Geometry: final body of the model. Coordinates: model frame, mm. Face numbers are marked on the shaded views. A direction names the side the tool comes from. Round coordinates to 2 decimals unless told otherwise and drop trailing zeros. Loops run counter-clockwise (first coordinate to the right, second up) from the corner with the lowest first, then second, coordinate; pieces in that order, holes last. Notation, with made-up numbers: (19.25, -37.75) - (50.25, -37.75) arc R16 cw to (50.25, -11.75) - close; hole circle Ø3 at (59.5, 2.5). An arc over 180 degrees is marked (long way). Answer as a JSON object with one key per item and string values. Group by question number.
Item 1: Section C-C (x = 111). Return the cut outline in (y, z), plus the area to 3 significant figures.
Item 2: Reachability of the marked faces 1 and 2 from +Z, -Z, +X, -X, +Y, -Y: full face, straight path, thin tool, end or side. Return the list, or none.
Item 3: Section D-D (y = 41). Return the cut outline in (x, z), plus the area to 3 significant figures.
Item 4: Section B-B (y = 10.5). Return the cut outline in (x, z), plus the area to 3 significant figures.
Item 5: Draft query along X for the marked faces 3, 4, 5 and 6. Return one class per face: released by +X, released by -X, zero draft, split by the parting line, or undercut.
Item 6: Line query: line 1 (Z direction, x = 30, y = 2); line 2 (Y direction, x = 100.5, z = 15.5); line 3 (X direction, y = 50, z = 6.5). Output: solid intervals per line, ascending.
Item 7: Section A-A (z = 10). Return the cut outline in (x, y).
Item 8: First-contact query: pin 1 (1.6 mm diameter, centred on x = 36, z = 15, fed in from +Y); pin 2 (2 mm diameter, centred on x = 115, y = 55.5, fed in from +Z); pin 3 (3 mm diameter, centred on x = 36, z = 15, fed in from -Y). Flat tips, straight axial feed; report the tip coordinate or a pass-through.
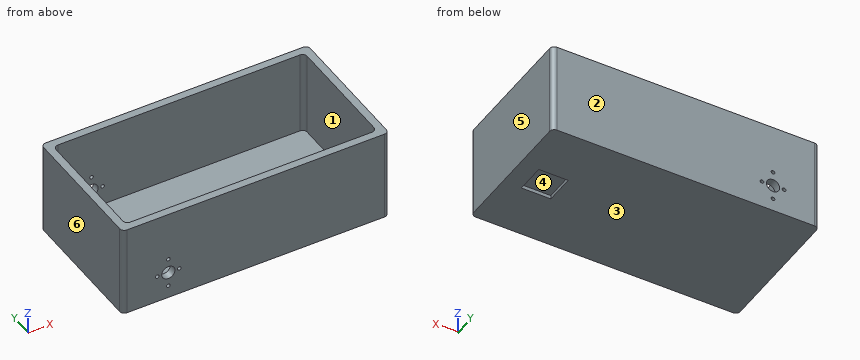
Autodesk Fusion 360 part; units mm, degrees
sketch "Skizze1" plane through (0, 0, 0) normal (0, 0, 1) x (1, 0, 0)
  line L0 (5, 0) -> (150, 0)
  line L1 (150, 0) -> (150, 75)
  line L2 (150, 75) -> (5, 75)
  line L3 (5, 75) -> (5, 0)
extrude "Extrusion1" add sketch "Skizze1" along normal blind 50
shell "Schale1" thickness 4.2 removed faces 1 at (53.3333, 50, 50)
fillet "Abrundung1" radius 2.5 1 edges at (5, 0, 25)
fillet "Abrundung2" radius 2.5 1 edges at (9.2, 4.2, 27.1)
fillet "Abrundung3" radius 2.5 1 edges at (9.2, 70.8, 27.1)
fillet "Abrundung4" radius 2.5 1 edges at (5, 75, 25)
fillet "Abrundung5" radius 2.5 1 edges at (150, 75, 25)
fillet "Abrundung6" radius 2.5 1 edges at (145.8, 70.8, 27.1)
fillet "Abrundung7" radius 2.5 1 edges at (145.8, 4.2, 27.1)
fillet "Abrundung8" radius 2.5 1 edges at (150, 0, 25)
sketch "Skizze2" plane through (0, 75, 0) normal (0, 1, 0) x (-1, 0, 0)
  line L0 (-147.5, 50) -> (-147.5, 0)
  line L1 (-147.5, 0) -> (-7.5, 0)
  line L2 (-7.5, 0) -> (-7.5, 50)
  line L3 (-7.5, 50) -> (-147.5, 50)
  circle A0 centre (-30, 7) radius 1
  dimension "d20" = 2
extrude "Extrusion2" cut sketch "Skizze2" against normal blind 300 contours A0
sketch "Skizze3" plane through (0, 75, 0) normal (0, 1, 0) x (-1, 0, 0)
  circle A0 centre (-30, 7) radius 1
  line L0 (-147.5, 50) -> (-147.5, 0)
  line L1 (-147.5, 0) -> (-7.5, 0)
  line L2 (-7.5, 0) -> (-7.5, 50)
  line L3 (-7.5, 50) -> (-147.5, 50)
  circle A1 centre (-30, 23) radius 1
  dimension "d23" = 2
extrude "Extrusion3" cut sketch "Skizze3" against normal blind 300 contours A1
sketch "Skizze4" plane through (0, 75, 0) normal (0, 1, 0) x (-1, 0, 0)
  circle A0 centre (-30, 23) radius 1
  circle A1 centre (-30, 7) radius 1
  line L0 (-147.5, 50) -> (-147.5, 0)
  line L1 (-147.5, 0) -> (-7.5, 0)
  line L2 (-7.5, 0) -> (-7.5, 50)
  line L3 (-7.5, 50) -> (-147.5, 50)
  circle A2 centre (-24, 15) radius 1
  circle A3 centre (-36, 15) radius 1
  dimension "d26" = 2
  dimension "d27" = 2
extrude "Extrusion4" cut sketch "Skizze4" against normal blind 300 contours A2
sketch "Skizze5" plane through (0, 75, 0) normal (0, 1, 0) x (-1, 0, 0)
  circle A0 centre (-24, 15) radius 1
  circle A1 centre (-30, 23) radius 1
  circle A2 centre (-30, 7) radius 1
  line L0 (-147.5, 50) -> (-147.5, 0)
  line L1 (-147.5, 0) -> (-7.5, 0)
  line L2 (-7.5, 0) -> (-7.5, 50)
  line L3 (-7.5, 50) -> (-147.5, 50)
  circle A3 centre (-36, 15) radius 1
  dimension "d30" = 2
extrude "Extrusion5" cut sketch "Skizze5" against normal blind 300 contours A3
sketch "Skizze6" plane through (0, 75, 0) normal (0, 1, 0) x (-1, 0, 0)
  circle A0 centre (-36, 15) radius 1
  circle A1 centre (-24, 15) radius 1
  circle A2 centre (-30, 23) radius 1
  circle A3 centre (-30, 7) radius 1
  line L0 (-147.5, 50) -> (-147.5, 0)
  line L1 (-147.5, 0) -> (-7.5, 0)
  line L2 (-7.5, 0) -> (-7.5, 50)
  line L3 (-7.5, 50) -> (-147.5, 50)
  circle A4 centre (-30, 15) radius 3.6
  dimension "d33" = 7.2
extrude "Extrusion6" cut sketch "Skizze6" against normal blind 300 contours A4
sketch "Skizze7" plane through (0, 0, 0) normal (0, 0, -1) x (1, 0, 0)
  arc A0 (150, -2.5) -> (147.5, 0) centre (147.5, -2.5) ccw
  line L0 (147.5, 0) -> (7.5, 0)
  arc A1 (7.5, 0) -> (5, -2.5) centre (7.5, -2.5) ccw
  line L1 (5, -2.5) -> (5, -72.5)
  arc A2 (5, -72.5) -> (7.5, -75) centre (7.5, -72.5) ccw
  line L2 (7.5, -75) -> (147.5, -75)
  arc A3 (147.5, -75) -> (150, -72.5) centre (147.5, -72.5) ccw
  line L3 (150, -72.5) -> (150, -2.5)
  line L4 (140, -29.5) -> (124, -29.5)
  line L5 (124, -29.5) -> (124, -45.5)
  line L6 (124, -45.5) -> (140, -45.5)
  line L7 (140, -45.5) -> (140, -29.5)
extrude "Extrusion7" cut sketch "Skizze7" against normal blind 2 contours L4 L5 L6 L7
Values:
{
 "1": {"outline": "(0, 0) - (75, 0) - (75, 50) - (70.8, 50) - (70.8, 4.2) - (4.2, 4.2) - (4.2, 50) - (0, 50) - close", "area": "700 mm^2"},
 "2": {"face 1": "+Z", "face 2": "+Z, -Z, +X, -X, +Y"},
 "3": {"outline": "(5, 0) - (124, 0) - (124, 2) - (140, 2) - (140, 0) - (150, 0) - (150, 50) - (145.8, 50) - (145.8, 4.2) - (9.2, 4.2) - (9.2, 50) - (5, 50) - close", "area": "962 mm^2"},
 "4": {"outline": "(5, 0) - (150, 0) - (150, 50) - (145.8, 50) - (145.8, 4.2) - (9.2, 4.2) - (9.2, 50) - (5, 50) - close", "area": "994 mm^2"},
 "5": {"face 3": "zero draft", "face 4": "undercut", "face 5": "released by +X", "face 6": "released by -X"},
 "6": {"line 1": "z = 0 to 6, 8 to 11.4, 18.6 to 22, 24 to 50", "line 2": "y = 0 to 4.2, 70.8 to 75", "line 3": "x = 5 to 9.2, 145.8 to 150"},
 "7": {"outline": "(5, 2.5) arc R2.5 ccw to (7.5, 0) - (147.5, 0) arc R2.5 ccw to (150, 2.5) - (150, 72.5) arc R2.5 ccw to (147.5, 75) - (7.5, 75) arc R2.5 ccw to (5, 72.5) - close; hole (9.2, 6.7) arc R2.5 ccw to (11.7, 4.2) - (143.3, 4.2) arc R2.5 ccw to (145.8, 6.7) - (145.8, 68.3) arc R2.5 ccw to (143.3, 70.8) - (11.7, 70.8) arc R2.5 ccw to (9.2, 68.3) - close"},
 "8": {"pin 1": "passes through", "pin 2": "stops at z = 4.2", "pin 3": "stops at y = 0"}
}
